Autodesk Inventor part; units mm, degrees
ref_plane "YZ Plane" through (0, 0, 0) normal (1, 0, 0) x (0, 1, 0)
ref_plane "XZ Plane" through (0, 0, 0) normal (0, 1, 0) x (-1, 0, 0)
ref_plane "XY Plane" through (0, 0, 0) normal (0, 0, 1) x (1, 0, 0)
sketch "Sketch1" plane through (0, 0, 0) normal (0, 0, 1) x (1, 0, 0)
  line L0 (-50.0126, 6.35) -> (50.0126, 6.35)
  line L1 (50.0126, 6.35) -> (50.0126, -6.35)
  line L2 (50.0126, -6.35) -> (-50.0126, -6.35)
  line L3 (-50.0126, -6.35) -> (-50.0126, 6.35)
  line L4 (-50.0126, 6.35) -> (50.0126, -6.35) construction
  line L5 (50.0126, 6.35) -> (-50.0126, -6.35) construction
  point P0 (0, 0)
  dimension "d0" = 100.0252
  dimension "d1" = 12.7
extrude "Extrusion1" add sketch "Sketch1" along normal blind 25.4
sketch "Sketch2" plane through (0, 0, 0) normal (0, 0, 1) x (1, 0, 0)
  line L0 (-50.0126, -6.35) -> (50.0126, -6.35)
  line L1 (-50.0126, 6.35) -> (-50.0126, -6.35)
  line L2 (50.0126, 6.35) -> (-50.0126, 6.35)
  line L3 (50.0126, -6.35) -> (50.0126, 6.35)
  line L4 (-70.0176, 0) -> (70.0176, 0)
  line L5 (0, -8.89) -> (0, 8.89)
  line L6 (50.0126, -6.35) -> (50.0126, 6.35)
  line L7 (-50.0126, -6.35) -> (50.0126, -6.35)
  line L8 (50.0126, 6.35) -> (38.3286, 6.35)
  line L9 (38.3286, 6.35) -> (38.3286, -6.35)
  line L10 (38.3286, -6.35) -> (50.0126, -6.35)
  line L11 (50.0126, -6.35) -> (50.0126, 6.35)
  point P0 (0, 0)
  point P1 (38.3286, 6.35)
  point P2 (38.3286, -6.35)
  dimension "d4" = 11.684
extrude "Extrusion2" add sketch "Sketch2" against normal blind 12.7 contours L9 L4 L3 L0 | L9 L2 L3 L4
mirror "Mirror1" about plane through (0, 0, 0) normal (1, 0, 0) of "Extrusion2"
fillet "Fillet1" radius 3.175 2 edges at (38.3286, 0, 0) (-38.3286, 0, 0)
sketch "Sketch3" plane through (0, 0, 0) normal (0, 0, -1) x (-1, 0, 0)
  line L0 (70.0176, 0) -> (-70.0176, 0)
  line L1 (0, -8.89) -> (0, 8.89)
  line L2 (35.1536, 6.35) -> (35.1536, -6.35)
  line L3 (-35.1536, 6.35) -> (35.1536, 6.35)
  line L4 (-35.1536, -6.35) -> (-35.1536, 6.35)
  line L5 (35.1536, -6.35) -> (-35.1536, -6.35)
  circle A0 centre (0, -4.1402) radius 2.0574
  point P0 (0, 0)
  dimension "d9" = 4.1148
  dimension "d10" = 2.2098
extrude "Extrusion3" cut sketch "Sketch3" against normal blind 1.5875 contours A0 L1 | L1 A0
pattern_linear "Rectangular Pattern1" count 11 spacing 6.35 along (1, 0, 0) of "Extrusion3" first direction both ways yes
sketch "Sketch4" plane through (0, 0, -12.7) normal (0, 0, -1) x (-1, 0, 0)
  line L0 (70.0176, 0) -> (-70.0176, 0)
  line L1 (0, -8.89) -> (0, 8.89)
  line L2 (-50.0126, -6.35) -> (-38.3286, -6.35)
  line L3 (-38.3286, -6.35) -> (-38.3286, 6.35)
  line L4 (-38.3286, 6.35) -> (-50.0126, 6.35)
  line L5 (-50.0126, 6.35) -> (-50.0126, -6.35)
  line L6 (50.0126, -6.35) -> (38.3286, -6.35)
  line L7 (50.0126, 6.35) -> (50.0126, -6.35)
  line L8 (38.3286, 6.35) -> (50.0126, 6.35)
  line L9 (38.3286, -6.35) -> (38.3286, 6.35)
  line L10 (-38.3286, -6.35) -> (-38.3286, 6.35)
  line L11 (-38.3286, 3.683) -> (-39.3446, 3.683)
  line L12 (-39.3446, 3.683) -> (-39.3446, -5.842)
  line L13 (-39.3446, -5.842) -> (-38.3286, -5.842)
  line L14 (-38.3286, -5.842) -> (-38.3286, 3.683)
  point P0 (0, 0)
  point P1 (-38.3286, 3.683)
  dimension "d19" = 1.016
  dimension "d20" = 9.525
  dimension "d21" = 0.508
extrude "Extrusion4" cut sketch "Sketch4" against normal blind 6.35 contours L3 L13 L12 L0 | L0 L12 L11 L3
mirror "Mirror2" about plane through (0, 0, 0) normal (1, 0, 0) of "Extrusion4"
sketch "Sketch5" plane through (0, 0, -12.7) normal (0, 0, -1) x (-1, 0, 0)
  line L0 (-38.3286, -5.842) -> (-39.3446, -5.842)
  line L1 (-39.3446, -5.842) -> (-39.3446, 3.683)
  line L2 (-39.3446, 3.683) -> (-38.3286, 3.683)
  line L3 (-38.3286, 3.683) -> (-38.3286, 6.35)
  line L4 (-38.3286, 6.35) -> (-50.0126, 6.35)
  line L5 (-50.0126, 6.35) -> (-50.0126, -6.35)
  line L6 (-50.0126, -6.35) -> (-38.3286, -6.35)
  line L7 (-38.3286, -6.35) -> (-38.3286, -5.842)
  line L8 (47.9806, -6.35) -> (47.9806, 6.35)
  line L9 (50.0126, 6.35) -> (50.0126, -6.35)
  line L10 (38.3286, 3.683) -> (39.3446, 3.683)
  line L11 (39.3446, 3.683) -> (39.3446, -5.842)
  line L12 (39.3446, -5.842) -> (38.3286, -5.842)
  line L13 (38.3286, -6.35) -> (38.3286, -5.842)
  line L14 (50.0126, -6.35) -> (38.3286, -6.35)
  line L15 (50.0126, 6.35) -> (50.0126, -6.35)
  line L16 (38.3286, 6.35) -> (50.0126, 6.35)
  line L17 (38.3286, 3.683) -> (38.3286, 6.35)
  line L18 (70.0176, 0) -> (-70.0176, 0)
  line L19 (0, -8.89) -> (0, 8.89)
  circle A0 centre (-44.0182, 0.6604) radius 3.3782
  point P0 (0, 0)
  dimension "d24" = 6.7564
  dimension "d25" = 7.0104
  dimension "d26" = 5.9944
hole "Hole1" at (44.0182, 0.6604, -12.7) direction (0, 0, 1) diameter 4.9276 end through all
mirror "Mirror3" about plane through (0, 0, 0) normal (1, 0, 0) of "Hole1"
sketch "Sketch6" plane through (38.3286, 6.35, -12.7) normal (0, 1, 0) x (1, 0, 0)
  line L0 (11.684, -38.1) -> (-88.3412, -38.1)
  line L1 (11.684, 0) -> (11.684, -38.1)
  line L2 (0, 0) -> (11.684, 0)
  line L3 (0, -9.525) -> (0, 0)
  arc A0 (-3.175, -12.7) -> (0, -9.525) centre (-3.175, -9.525) ccw
  line L4 (-3.175, -12.7) -> (-73.4822, -12.7)
  arc A1 (-76.6572, -9.525) -> (-73.4822, -12.7) centre (-73.4822, -9.525) ccw
  line L5 (-76.6572, -9.525) -> (-76.6572, 0)
  line L6 (-76.6572, 0) -> (-88.3412, 0)
  line L7 (-88.3412, 0) -> (-88.3412, -38.1)
  line L8 (-108.397, -12.7) -> (31.9938, -12.7)
  line L9 (-38.3286, 7.62) -> (-38.3286, -45.72)
  line L10 (0, -9.525) -> (0, 0)
  line L11 (0, 0) -> (11.684, 0)
  line L12 (11.684, 0) -> (11.684, -38.1)
  line L13 (11.684, -38.1) -> (0, -38.1)
  line L14 (0, -38.1) -> (0, 0)
  line L15 (-88.3412, 0) -> (-88.3412, -38.1)
  line L16 (-76.6572, 0) -> (-88.3412, 0)
  line L17 (-76.6572, -9.525) -> (-76.6572, 0)
  arc A2 (-76.6572, -9.525) -> (-73.4822, -12.7) centre (-73.4822, -9.525) ccw
  line L18 (-76.6572, -9.525) -> (-76.6572, 0)
  line L19 (-76.6572, 0) -> (-88.3412, 0)
  line L20 (-88.3412, 0) -> (-88.3412, -38.1)
  line L21 (-88.3412, -38.1) -> (-76.6572, -38.1)
  line L22 (-76.6572, -38.1) -> (-76.6572, 0)
  point P0 (-38.3286, -12.7)
extrude "Extrusion5" add sketch "Sketch6" along normal blind 25.4 contours L0 L14 L8 L1 | L8 L14 L3 L2 L1 | L0 L7 L8 L22 | L8 L7 L6 L5 L22
chamfer "Chamfer2" distance 25.4 angle 45 2 edges at (44.1706, 31.75, 25.4) (-44.1706, 31.75, 25.4)
fillet "Fillet3" radius 12.7 2 edges at (38.3286, 6.35, 11.1125) (-38.3286, 6.35, 11.1125)
equation "\"d32\" = Thickness"
equation "\"BendRadius\" = Thickness"
equation "\"BendReliefWidth\" = Thickness"
equation "\"BendReliefDepth\" = 0.5 * Thickness"
equation "\"CornerReliefSize\" = 4 * Thickness"
equation "\"MinimumRemnant\" = 2 * Thickness"
equation "\"TransitionRadius\" = BendRadius"
equation "\"JacobiRadiusSize\" = BendRadius"
equation "\"GapSize\" = Thickness"
properties part number "_3DPrint"
For this review, take the finished solid that the model builds, in its own axes (mm). A direction names the side the tool comes from. Coordinates: 2 decimals unless noted, no trailing zeros. Order: outer loops, then holes, each group sorted by start corner. A loop starts at its lowest first (then second) coordinate and runs counter-clockwise, first axis right, second up. Notation, with made-up numbers: (-3, 8) - (35, 8) arc R26 ccw to (35, 44) - close; hole circle Ø2 at (77.5, 55). An arc over 180 degrees is marked (long way). Use one line per item in the form item = value.
Q1. Consider section A-A (y = 25.5). Give the boundary of the cut face in (x, z), then the cut area to 3 significant figures.
Checked values:
outline = (-50.01, -12.7) - (-38.33, -12.7) - (-38.33, 6.25) - (-50.01, 6.25) - close; (38.33, -12.7) - (50.01, -12.7) - (50.01, 6.25) - (38.33, 6.25) - close
area = 443 mm2
Q2. Consider section D-D (z = 10.5). Give the boundary of the cut face in (x, y).
Checked values:
outline = (-50.01, -6.35) - (50.01, -6.35) - (50.01, 21.25) - (38.33, 21.25) - (38.33, 19.05) arc R12.7 cw to (25.63, 6.35) - (-25.63, 6.35) arc R12.7 cw to (-38.33, 19.05) - (-38.33, 21.25) - (-50.01, 21.25) - close; hole circle Ø4.93 at (-44.02, 0.66); hole circle Ø4.93 at (44.02, 0.66)
Q3. For P1, Ø6.5, axis at x = -19.05, y = -4.14, coming from the -Z side; P2, Ø3.5, axis at x = 12.7, y = -4.14, coming from the -Z side; P3, Ø4, axis at x = -17.5, z = 10, coming from the +Y side, all flat-tipped, find the tip position at first contact; note any pin that passes through.
Checked values:
P1 = 0
P2 = 1.59
P3 = 6.35
Q4. For faces 1 (the cylindrical face through (21.105, -4.05, 0.783)), 2 (the flat face through (43.07, 19.23, 12.52)), 3 (the flat face through (-38.329, 17, -5)), 4 (the flat face through (0, 6.35, 13)), 5 (the flat face through (50.013, 9, 2)), list the 3-axis set-ups (+Z, -Z, +X, -X, +Y, -Y) from which the entire face can be reached by the end or side of a thin tool; tool diameter is ignored.
Checked values:
face_1 = -Z
face_2 = +Z, +X, -X, +Y
face_3 = -Z, +Y
face_4 = +Z, -Z, +Y
face_5 = +Z, -Z, +X, +Y, -Y
Q5. Draft analysis for pull direction X (two halves, no side actions). For faces 6 (the cylindrical face through (-8.31, -3.52, 0.78)), 7 (the flat face through (-44, 31.75, -6)), 8 (the flat face through (-50.013, 8, 2)), state which applies: +X half, -X half, draft (parallel to the pull), parting line (faces both ways), or undercut.
Checked values:
face_6 = undercut
face_7 = draft
face_8 = -X half
Q6. For probe 1 along Y at (x, z) = (-12.7, 1); probe 2 along X at (y, z) = (23, 1); probe 3 along Z at (x, y) = (-31.5, 1), list the stretches that pass through material, from the lowest coordinate up. Write a range as from..to.
Checked values:
probe_1 = -6.35..-6.2, -2.08..6.35
probe_2 = -50.01..-38.33, 38.33..50.01
probe_3 = 0..25.4
Q7. Consider section C-C (x = 6.35). Give the boundary of the cut face in (y, z), then the cut area to 3 significant figures.
Checked values:
outline = (-6.35, 0) - (-6.2, 0) - (-6.2, 1.59) - (-2.08, 1.59) - (-2.08, 0) - (6.35, 0) - (6.35, 25.4) - (-6.35, 25.4) - close
area = 316 mm2
Q8. Consider section B-B (z = -7.5). Give the boundary of the cut face in (x, y).
Checked values:
outline = (-50.01, -6.35) - (-38.33, -6.35) - (-38.33, -5.84) - (-39.34, -5.84) - (-39.34, 3.68) - (-38.33, 3.68) - (-38.33, 31.75) - (-50.01, 31.75) - close; (38.33, -6.35) - (50.01, -6.35) - (50.01, 31.75) - (38.33, 31.75) - (38.33, 3.68) - (39.34, 3.68) - (39.34, -5.84) - (38.33, -5.84) - close; hole circle Ø4.93 at (-44.02, 0.66); hole circle Ø4.93 at (44.02, 0.66)
